```python
from build123d import *
from OCP.BRepFilletAPI import BRepFilletAPI_MakeChamfer

# Parameters (mm, degrees)
SKETCH_1_W                = 17
SKETCH_1_H                = 70
SKETCH_2_R                = 62.5
EXTRUDE_1_DEPTH           = 24
SKETCH_3_R                = 50
EXTRUDE_2_DEPTH           = 45
SKETCH_4_R                = 35
EXTRUDE_3_DEPTH           = 122
HOLE_WIZARD_3_D           = 8
HOLE_WIZARD_3_DEPTH       = 15
HOLE_WIZARD_3_CBORE_D     = 35
HOLE_WIZARD_3_CBORE_DEPTH = 5
HOLE_WIZARD_3_TIP         = 2.403442476
HOLE_WIZARD_5_D           = 8
HOLE_WIZARD_5_DEPTH       = 12
HOLE_WIZARD_5_CBORE_D     = 25
HOLE_WIZARD_5_CBORE_DEPTH = 2
HOLE_WIZARD_5_TIP         = 2.403442476
CHAMFER_2_SIZE            = 0.803847576
CHAMFER_2_SIZE2           = 3
CHAMFER_3_SIZE            = 0.999999999
CHAMFER_3_SIZE2           = 1.732050808
CHAMFER_4_SIZE            = 0.5
CHAMFER_5_SIZE            = 0.999999999
CHAMFER_5_SIZE2           = 1.000000001


with BuildPart() as part:
    # 草圖1 → 旋轉1 (revolve)
    with BuildSketch(Plane(origin=(0, 0, 0), x_dir=(-1, 0, 0), z_dir=(0, 0, -1)), mode=Mode.PRIVATE) as revolve_1_sk:
        with Locations((-32.5, 35)):
            Rectangle(SKETCH_1_W, SKETCH_1_H)
    revolve(revolve_1_sk.sketch.rotate(Axis((41, 0, 0), (-1, 0, 0)), 270), axis=Axis((41, 0, 0), (-1, 0, 0)))

    # 草圖2 → 填料-伸長1 (add)
    with BuildSketch(Plane.ZY.offset(-24)):
        Circle(SKETCH_2_R)
    extrude(amount=EXTRUDE_1_DEPTH)

    # 草圖3 → 填料-伸長2 (add)
    with BuildSketch(Plane(origin=(41, 0, 0), x_dir=(0, 0, -1), z_dir=(1, 0, 0))):
        with Locations(Location((0, 0, 0), (0, 0, 180))):
            Circle(SKETCH_3_R)
    extrude(amount=EXTRUDE_2_DEPTH)

    # 草圖4 → 填料-伸長3 (add)
    with BuildSketch(Plane(origin=(86, 0, 0), x_dir=(0, 0, -1), z_dir=(1, 0, 0))):
        with Locations(Location((0, 0, 0), (0, 0, 180))):
            Circle(SKETCH_4_R)
    extrude(amount=EXTRUDE_3_DEPTH)

    # 鑽孔3
    with Locations(Plane(origin=(208, 0, 0), x_dir=(0, 0, -1), z_dir=(1, 0, 0))):
        with Locations((0, 0)):
            CounterBoreHole(HOLE_WIZARD_3_D / 2, HOLE_WIZARD_3_CBORE_D / 2, HOLE_WIZARD_3_CBORE_DEPTH, depth=HOLE_WIZARD_3_DEPTH)
            with Locations((0, 0, -(HOLE_WIZARD_3_DEPTH + HOLE_WIZARD_3_TIP / 2))):  # 118° drill point
                Cone(0, HOLE_WIZARD_3_D / 2, HOLE_WIZARD_3_TIP, mode=Mode.SUBTRACT)

    # 鑽孔5
    with Locations(Plane.ZY):
        with Locations((0, 0)):
            CounterBoreHole(HOLE_WIZARD_5_D / 2, HOLE_WIZARD_5_CBORE_D / 2, HOLE_WIZARD_5_CBORE_DEPTH, depth=HOLE_WIZARD_5_DEPTH)
            with Locations((0, 0, -(HOLE_WIZARD_5_DEPTH + HOLE_WIZARD_5_TIP / 2))):  # 118° drill point
                Cone(0, HOLE_WIZARD_5_D / 2, HOLE_WIZARD_5_TIP, mode=Mode.SUBTRACT)

    # 導角2
    chamfer_2_edges = [part.edges().sort_by_distance(p)[0] for p in [
        (208, 0, -35),
    ]]
    chamfer_2_side = [part.faces().sort_by_distance(p)[0] for p in [
        (208, 0, -34.010050506),
    ]]
    chamfer(chamfer_2_edges, length=CHAMFER_2_SIZE, length2=CHAMFER_2_SIZE2, reference=chamfer_2_side[0])

    # 導角3: one chamfer whose edges measure the first distance from different faces: ONE call of the kernel's chamfer builder (chamfer() names one face for all edges)
    chamfer_3_edges_1 = [part.edges().sort_by_distance(p)[0] for p in [
        (203, 0, -4),
    ]]
    chamfer_3_side_1 = [part.faces().sort_by_distance(p)[0] for p in [
        (203, 0, 17.005025253),
    ]]
    chamfer_3_edges_2 = [part.edges().sort_by_distance(p)[0] for p in [
        (2, 0, 4),
    ]]
    chamfer_3_side_2 = [part.faces().sort_by_distance(p)[0] for p in [
        (2, 0, -12.146446609),
    ]]
    chamfer_3 = BRepFilletAPI_MakeChamfer(part.part.solid().wrapped)
    for e in chamfer_3_edges_1:
        chamfer_3.Add(CHAMFER_3_SIZE, CHAMFER_3_SIZE2, e.wrapped, chamfer_3_side_1[0].wrapped)  # the first distance lies on this face
    for e in chamfer_3_edges_2:
        chamfer_3.Add(CHAMFER_3_SIZE, CHAMFER_3_SIZE2, e.wrapped, chamfer_3_side_2[0].wrapped)  # the first distance lies on this face
    add(Compound.cast(chamfer_3.Shape()), mode=Mode.REPLACE)

    # 導角4
    chamfer_4_edges = [part.edges().sort_by_distance(p)[0] for p in [
        (86, 0, -50),
        (24, 0, -70),
        (41, 0, -70),
    ]]
    chamfer(chamfer_4_edges, length=CHAMFER_4_SIZE)

    # 導角5
    chamfer_5_edges = [part.edges().sort_by_distance(p)[0] for p in [
        (0, 0, -62.5),
    ]]
    chamfer_5_side = [part.faces().sort_by_distance(p)[0] for p in [
        (12, 0, -62.5),
    ]]
    chamfer(chamfer_5_edges, length=CHAMFER_5_SIZE, length2=CHAMFER_5_SIZE2, reference=chamfer_5_side[0])


solid = part.part
```
CAD build for the part. Positions are in the model's coordinates, mm. A direction names the side the tool comes from. Coordinates: 2 decimals unless noted, no trailing zeros. Order: outer loops, then holes, each group sorted by start corner. A loop starts at its lowest first (then second) coordinate and runs counter-clockwise, first axis right, second up. Notation, with made-up numbers: (-33.75, 35.5) - (-22.75, 35.5) arc R31 cw to (-22.75, 64.5) - close; hole circle Ø1 at (21.25, 57). An arc over 180 degrees is marked (long way). Answer in a Markdown table with one row per item.
1. Slice it at B-B, the plane x = 175. List the corners of the cut face in (y, z).
Answer:
| item | result |
|---|---|
| outline | circle Ø70 at (0, 0) |
2. Pull direction Y, two halves, no side cores. Call faces 1 (the face through (41, -45, -30)), 2 (the face through (207.812, 33.432, -7.424)), 3 (the face through (203, -4, -4)), 4 (the face through (0.986, 3.755, 11.923)): +Y half, -Y half, draft (parallel to the pull), parting line (faces both ways), or undercut.
Answer:
| item | result |
|---|---|
| face 1 | draft |
| face 2 | parting line |
| face 3 | undercut |
| face 4 | undercut |
3. Flat gauge pins, fed straight in: P1, Ø22.5, axis at y = 0, z = 0, coming from the -X side; P2, Ø3, axis at x = 63, y = 39, coming from the +Z side; P3, Ø1, axis at x = 27, z = 32.5, coming from the -Y side. Where does each tip first touch, or does it go through?
Answer:
| item | result |
|---|---|
| P1 | x = 2 |
| P2 | z = 33.07 |
| P3 | y = -62.26 |
4. Slice it at A-A, the plane x = 71.5. List the corners of the cut face in (y, z).
Answer:
| item | result |
|---|---|
| outline | circle Ø100 at (0, 0) |
5. 3-axis set-ups, long thin cutter, end or side, ignore diameter. For faces 5 (the face through (12.66, 2.75, -62.44)), 6 (the face through (0, -13, -1)), 7 (the face through (197.076, -3.905, -0.867)): which of +Z, -Z, +X, -X, +Y, -Y reach the whole face in a straight line?
Answer:
| item | result |
|---|---|
| face 5 | -X |
| face 6 | +Z, -Z, -X, +Y, -Y |
| face 7 | +X |
6. Drill centre lines: L1, parallel to Y at x = 204.2, z = 0; L2, parallel to Y at x = 1.35, z = 0; L3, parallel to X at y = -49.5, z = -43. Where is each one in solid material? Low to high. Write a range as from..to.
Answer:
| item | result |
|---|---|
| L1 | -35..-17.5, 17.5..35 |
| L2 | -62.5..-12.5, 12.5..62.5 |
| L3 | 24..41 |
